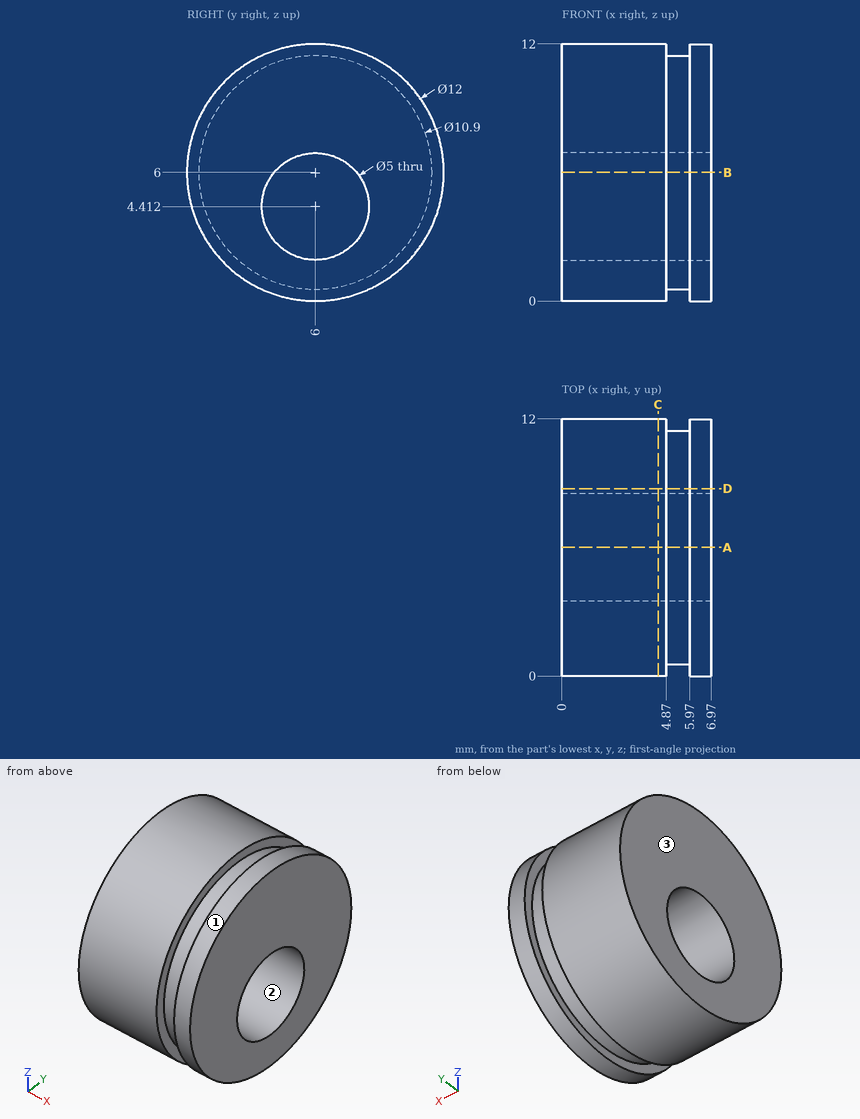
Verification items for this drawing (mm, ordinates from the low corner). Give positions to 0.01 mm unless a question says otherwise; leave off trailing zeros. Write each loop counter-clockwise with the first axis right and the second up, starting at its lowest first coordinate (ties: lowest second). Pieces come first, ordered by that corner, then holes.
1) Section check C-C, the plane x = 4.5. Record the boundary of the cut face in (y, z).
2) Section check D-D, the plane y = 8.75. Record the boundary of the cut face in (x, z) (1 decimal).
3) Section check B-B, the plane z = 6. Record the boundary of the cut face in (x, y).
4) Material ranges on L1, parallel to Z at x = 6, y = 6; L2, parallel to X at y = 11.25, z = 4; L3, parallel to Z at x = 5.25, y = 6, recorded low to high.
5) Section check A-A, the plane y = 6. Record the boundary of the cut face in (x, z).
6) Release check for a two-part mould opening along Y. For the marked faces 1, 2 and 3 record: pulls with the +Y half, pulls with the -Y half, needs draft (parallel to the pull), parting line crosses it, or undercut.
7) Gauge pin test, flat ends, axial feed: pin 1 (1.5 mm diameter, centred on x = 1.5, y = 9, fed in from -Z); pin 2 (2 mm diameter, centred on y = 5.5, z = 5, fed in from -X); pin 3 (4 mm diameter, centred on x = 1.5, z = 9, fed in from +Y). Record the tip position at first contact, or that the pin passes through.
Computed:
1. outline: circle Ø12 at (6, 6); hole circle Ø5 at (6, 4.41)
2. outline: (0, 0.7) - (4.9, 0.7) - (4.9, 1.3) - (6, 1.3) - (6, 0.7) - (7, 0.7) - (7, 11.3) - (6, 11.3) - (6, 10.7) - (4.9, 10.7) - (4.9, 11.3) - (0, 11.3) - close
3. outline: (0, 0) - (4.87, 0) - (4.87, 0.55) - (5.97, 0.55) - (5.97, 0) - (6.97, 0) - (6.97, 4.07) - (0, 4.07) - close; (0, 7.93) - (6.97, 7.93) - (6.97, 12) - (5.97, 12) - (5.97, 11.45) - (4.87, 11.45) - (4.87, 12) - (0, 12) - close
4. L1: z = 0 to 1.91, 6.91 to 12
4. L2: x = 0 to 4.87, 5.97 to 6.97
4. L3: z = 0.55 to 1.91, 6.91 to 11.45
5. outline: (0, 0) - (4.87, 0) - (4.87, 0.55) - (5.97, 0.55) - (5.97, 0) - (6.97, 0) - (6.97, 1.91) - (0, 1.91) - close; (0, 6.91) - (6.97, 6.91) - (6.97, 12) - (5.97, 12) - (5.97, 11.45) - (4.87, 11.45) - (4.87, 12) - (0, 12) - close
6. face 1: parting line crosses it
6. face 2: undercut
6. face 3: needs draft
7. pin 1: stops at z = 0.44
7. pin 2: passes through
7. pin 3: stops at y = 11.92
